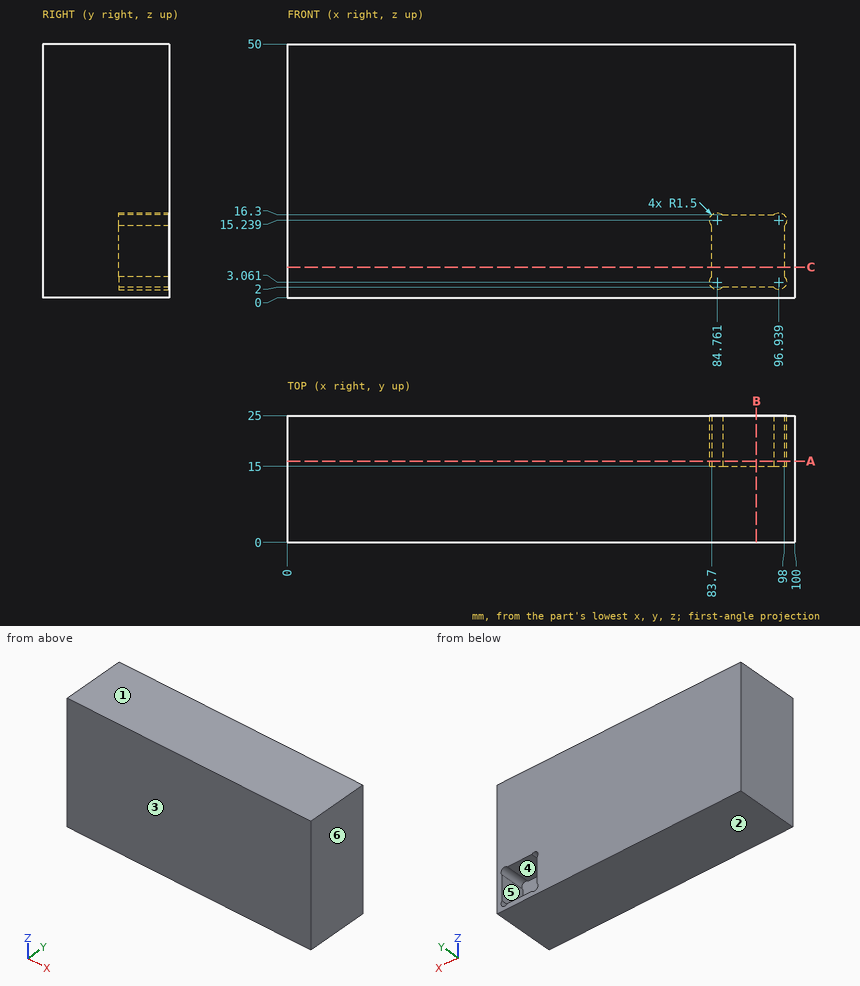
Design review of the part shown in the three views and the two pictorial views. Dimensions are in mm from the part's minimum x, y and z. A direction names the side the tool comes from. Give positions to 0.01 mm unless a question says otherwise; leave off trailing zeros. Write each loop counter-clockwise with the first axis right and the second up, starting at its lowest first coordinate (ties: lowest second). Pieces come first, ordered by that corner, then holes. Notation, with made-up numbers: (6.25, 74) -> (65.25, 74) arc R28 ccw to (65.25, 95) -> close; hole circle Ø3 at (70.5, 78.5). An arc over 180 degrees is marked (long way). Answer in a Markdown table with one row per item.
1) Tool access review of the marked faces 5 and 6: name each direction out of +Z, -Z, +X, -X, +Y, -Y from which nothing blocks a thin tool from reaching the whole face with its end or side.
Worked answers:
| item | result |
|---|---|
| face 5 | +Y |
| face 6 | +Z, -Z, +X, +Y, -Y |
2) Mouldability with a two-part tool opening along Z and no side actions: class the marked faces 1, 2, 3 and 4 as +Z half, -Z half, draft (parallel to the pull), parting line (faces both ways), or undercut.
Worked answers:
| item | result |
|---|---|
| face 1 | +Z half |
| face 2 | -Z half |
| face 3 | draft |
| face 4 | undercut |
3) Add section B-B on x = 92.5. State the section outline as (y, z) points, plus the area to 3 significant figures.
Worked answers:
| item | result |
|---|---|
| outline | (0, 0) -> (25, 0) -> (25, 2) -> (15, 2) -> (15, 16.3) -> (25, 16.3) -> (25, 50) -> (0, 50) -> close |
| area | 1,110 mm² |
4) For L1, parallel to Z at x = 88, y = 19.75; L2, parallel to Y at x = 87.5, z = 6; L3, parallel to X at y = 20.75, z = 2.5, list the stretches that pass through material, from the lowest coordinate up. Write a range as [from, to].
Worked answers:
| item | result |
|---|---|
| L1 | [0, 2], [16.3, 50] |
| L2 | [0, 15] |
| L3 | [0, 83.37], [98.33, 100] |
5) Add section C-C on z = 6. State the section outline as (x, y) points.
Worked answers:
| item | result |
|---|---|
| outline | (0, 0) -> (100, 0) -> (100, 25) -> (98, 25) -> (98, 15) -> (83.7, 15) -> (83.7, 25) -> (0, 25) -> close |
6) Add section A-A on y = 16. State the section outline as (x, z) points, plus the area to 3 significant figures.
Worked answers:
| item | result |
|---|---|
| outline | (0, 0) -> (100, 0) -> (100, 50) -> (0, 50) -> close; hole (83.7, 4.12) arc R1.5 ccw to (85.82, 2) -> (95.88, 2) arc R1.5 ccw to (98, 4.12) -> (98, 14.18) arc R1.5 ccw to (95.88, 16.3) -> (85.82, 16.3) arc R1.5 ccw to (83.7, 14.18) -> close |
| area | 4,790 mm² |
